Design review of the part built by this model. Coordinates are the model's own, in mm. Face numbers are marked on the shaded views. A direction names the side the tool comes from. Give positions to 0.01 mm unless a question says otherwise; leave off trailing zeros. Order: outer loops, then holes, each group sorted by start corner. A loop starts at its lowest first (then second) coordinate and runs counter-clockwise, first axis right, second up. Notation, with made-up numbers: M -36,19.25 L 22,19.25 A12 ccw 22,33.25 Z; hole C 82.25,-38 d11. An arc over 180 degrees is marked long. Put each result on its own line as item: value. Start each with the question number.
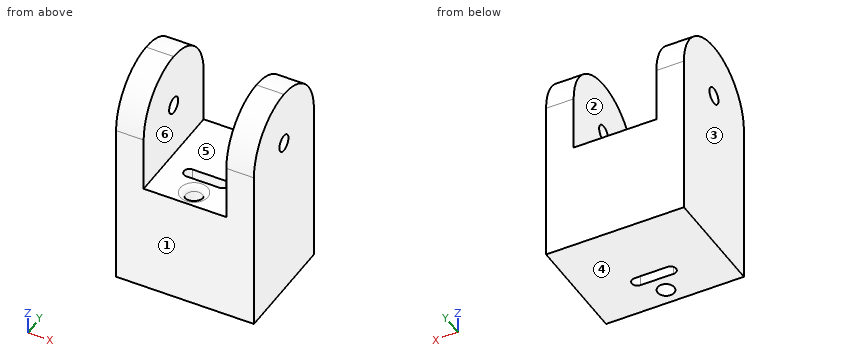
from build123d import *

# Parameters (mm, degrees)
SKETCH1_W           = 25
SKETCH1_H           = 20
BOSS_EXTRUDE1_DEPTH = 40
SKETCH2_W           = 15
SKETCH2_H           = 20
CUT_EXTRUDE1_DEPTH  = 20
SKETCH3_R           = 1.5
CUT_EXTRUDE2_DEPTH  = 30
FILLET1_R           = 10
SKETCH4_R           = 1.5
CUT_EXTRUDE3_DEPTH  = 20
FILLET2_R           = 1
CUT_EXTRUDE4_DEPTH  = 20


with BuildPart() as part:
    # Sketch1 → Boss-Extrude1 (new body)
    with BuildSketch(Plane.XY):
        Rectangle(SKETCH1_W, SKETCH1_H)
    extrude(amount=BOSS_EXTRUDE1_DEPTH)

    # Sketch2 → Cut-Extrude1 (cut)
    with BuildSketch(Plane.XY.offset(40)):
        Rectangle(SKETCH2_W, SKETCH2_H)
    extrude(amount=-CUT_EXTRUDE1_DEPTH, mode=Mode.SUBTRACT)

    # Sketch3 → Cut-Extrude2 (cut)
    with BuildSketch(Plane(origin=(12.5, 0, 0), x_dir=(0, 0, -1), z_dir=(1, 0, 0))):
        with Locations(Location((-30, 0, 0), (0, 0, 90))):
            Circle(SKETCH3_R)
    extrude(amount=-CUT_EXTRUDE2_DEPTH, mode=Mode.SUBTRACT)

    # Fillet1
    fillet1_edges = [part.edges().sort_by_distance(p)[0] for p in [
        (-10, 10, 40),
        (10, 10, 40),
        (10, -10, 40),
        (-10, -10, 40),
    ]]
    fillet(fillet1_edges, radius=FILLET1_R - 0.0001)  # a hair under: the kernel refuses the full size

    # Sketch4 → Cut-Extrude3 (cut)
    with BuildSketch(Plane.XY.offset(20)):
        with Locations((0, -7)):
            Circle(SKETCH4_R)
    extrude(amount=-CUT_EXTRUDE3_DEPTH, mode=Mode.SUBTRACT)

    # Fillet2
    fillet2_edges = [part.edges().sort_by_distance(p)[0] for p in [
        (-1.5, -7, 20),
    ]]
    fillet(fillet2_edges, radius=FILLET2_R)

    # Sketch5 → Cut-Extrude4 (cut)
    with BuildSketch(Plane.XY.offset(20)):
        with BuildLine():
            Line((-3, -2), (3, -2))
            ThreePointArc((3, -2), (4, -3), (3, -4))
            Line((3, -4), (-3, -4))
            ThreePointArc((-3, -4), (-4, -3), (-3, -2))
        make_face()
    extrude(amount=-CUT_EXTRUDE4_DEPTH, mode=Mode.SUBTRACT)


solid = part.part
1. Consider section B-B on z = 26. Give the boundary of the cut face in (x, y), then the cut area to 3 significant figures.
2. To check wall thickness, follow probe 1 along Y at (x, z) = (0, 8); probe 2 along Z at (x, y) = (-10.4, 0); probe 3 along X at (y, z) = (7.25, 35). State the ranges of each line that lie inside material, in increasing order.
3. Consider section D-D on z = 6. Give the boundary of the cut face in (x, y).
4. Machinability: for the marked faces 1 and 2, which of the approach directions +Z, -Z, +X, -X, +Y, -Y give a long, thin tool a straight path to every point of the face, cutting with its end or side? Answer none if there is none.
5. Consider section C-C on y = -3.5. Give the boundary of the cut face in (x, z), then the cut area to 3 significant figures.
6. The part is to be moulded in two halves that separate along X. For the marked faces 3, 4, 5 and 6, say which applies: +X half, -X half, draft (parallel to the pull), parting line (faces both ways), or undercut.
7. Insertion check: pin 1 (2.5 mm diameter, centred on y = 0, z = 30, fed in from -X); pin 2 (6 mm diameter, centred on x = -8.5, y = 6.5, fed in from +Z); pin 3 (4.5 mm diameter, centred on x = -0.5, y = -2, fed in from +Z); pin 4 (6 mm diameter, centred on x = -5, z = 32, fed in from -Y). Each pin has a flat end and moves straight along its axis. Give the tip position at first contact, or say it passes through.
8. Consider section A-A on x = 0. Give the boundary of the cut face in (y, z).
Returned:
1. outline: M -12.5,-10 L -7.5,-10 L -7.5,10 L -12.5,10 Z; M 7.5,-10 L 12.5,-10 L 12.5,10 L 7.5,10 Z
1. area: 200 mm2
2. probe 1: y = -10 to -8.5, -5.5 to -4, -2 to 10
2. probe 2: z = 0 to 28.5, 31.5 to 40
2. probe 3: x = -12.5 to -7.5, 7.5 to 12.5
3. outline: M -12.5,-10 L 12.5,-10 L 12.5,10 L -12.5,10 Z; hole M -3,-4 L 3,-4 A1 ccw 3,-2 L -3,-2 A1 ccw Z; hole C 0,-7 d3
4. face 1: +Z, -Z, +X, -X, -Y
4. face 2: +Z, +Y, -Y
5. outline: M -12.5,0 L -3.87,0 L -3.87,20 L -7.5,20 L -7.5,39.37 L -12.5,39.37 Z; M 3.87,0 L 12.5,0 L 12.5,39.37 L 7.5,39.37 L 7.5,20 L 3.87,20 Z
5. area: 539 mm2
6. face 3: -X half
6. face 4: draft
6. face 5: undercut
6. face 6: undercut
7. pin 1: passes through
7. pin 2: stops at z = 39.37
7. pin 3: stops at z = 20
7. pin 4: stops at y = -9.99
8. outline: M -10,0 L -8.5,0 L -8.5,19 A1 ccw -9.5,20 L -10,20 Z; M -5.5,0 L -4,0 L -4,20 L -4.5,20 A1 ccw -5.5,19 Z; M -2,0 L 10,0 L 10,20 L -2,20 Z
